from build123d import *

# Parameters (mm, degrees)
SKETCH1_W           = 8.3
SKETCH1_H           = 14.6
BOSS_EXTRUDE1_DEPTH = 1.5
SKETCH2_R           = 1.7
CUT_EXTRUDE1_DEPTH  = 1.5
SKETCH3_W           = 2.7
SKETCH3_H           = 3.5
BOSS_EXTRUDE3_DEPTH = 1.5


with BuildPart() as part:
    # Sketch1 → Boss-Extrude1 (new body)
    with BuildSketch(Plane.XY):
        with Locations((4.15, 7.3)):
            Rectangle(SKETCH1_W, SKETCH1_H)
    extrude(amount=BOSS_EXTRUDE1_DEPTH)

    # Sketch2 → Cut-Extrude1 (cut)
    with BuildSketch(Plane.XY.offset(1.5)):
        with Locations((4.15, 11.6)):
            Circle(SKETCH2_R)
    extrude(amount=-CUT_EXTRUDE1_DEPTH, mode=Mode.SUBTRACT)

    # Sketch3 → Boss-Extrude3 (add)
    with BuildSketch(Plane.XY.offset(1.5)):
        with Locations((4.15, 6.85)):
            Rectangle(SKETCH3_W, SKETCH3_H)
    extrude(amount=BOSS_EXTRUDE3_DEPTH)


solid = part.part
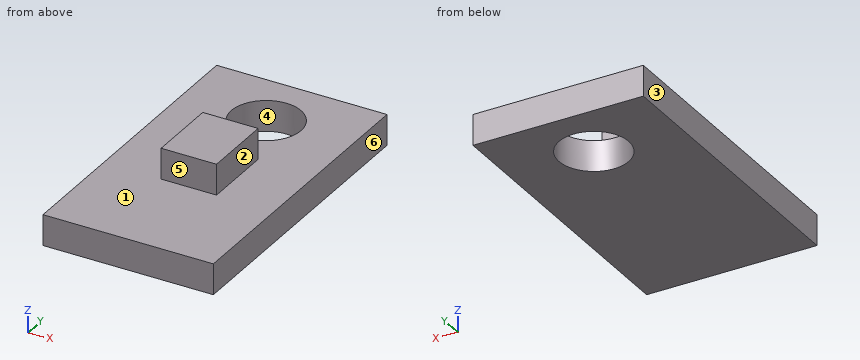
Verification items for the finished model (mm, model axes). Face numbers are marked on the shaded views. A direction names the side the tool comes from. Give positions to 0.01 mm unless a question says otherwise; leave off trailing zeros. Loops run counter-clockwise (first coordinate to the right, second up) from the corner with the lowest first, then second, coordinate; pieces in that order, holes last.
1) Thickness scan on line 1 along Y through (x, z) = (4.15, 0.9); line 2 along Z through (x, y) = (7.5, 3.25); line 3 along X through (y, z) = (7.25, 1.95). Record the ranges inside material, lowest first.
2) Sectioned sample at A-A, the plane x = 4.15. Enter the section's corners in (y, z), then the cut area to 4 significant figures.
3) Draft check along X on the marked faces 1, 2, 3 and 4. Enter one of: pulls with the +X half, pulls with the -X half, needs draft (parallel to the pull), parting line crosses it, or undercut.
4) Sectioned sample at C-C, the plane z = 0.8. Enter the section's corners in (x, y), then the cut area to 3 significant figures.
5) Set-up check for the marked faces 5 and 6: record each of +Z, -Z, +X, -X, +Y, -Y from which the full face is reachable in a straight line by a thin tool's end or side.
6) Sectioned sample at B-B, the plane y = 11.6. Enter the section's corners in (x, z), then the cut area to 3 significant figures.
7) Sectioned sample at D-D, the plane y = 8.25. Enter the section's corners in (x, z), then the cut area to 3 significant figures.
8) Depth check by flat-ended pin: pin 1 Ø1.5 at (x, z) = (2.5, 2.5) entering from -Y; pin 2 Ø1 at (x, y) = (4.5, 3) entering from +Z. Enter the tip coordinate at first touch or a pass-through.
Answers:
1. line 1: y = 0 to 9.9, 13.3 to 14.6
1. line 2: z = 0 to 1.5
1. line 3: x = 2.8 to 5.5
2. outline: (0, 0) - (9.9, 0) - (9.9, 1.5) - (8.6, 1.5) - (8.6, 3) - (5.1, 3) - (5.1, 1.5) - (0, 1.5) - close; (13.3, 0) - (14.6, 0) - (14.6, 1.5) - (13.3, 1.5) - close
2. area: 22.05 mm2
3. face 1: needs draft
3. face 2: pulls with the +X half
3. face 3: pulls with the -X half
3. face 4: undercut
4. outline: (0, 0) - (8.3, 0) - (8.3, 14.6) - (0, 14.6) - close; hole circle Ø3.4 at (4.15, 11.6)
4. area: 112 mm2
5. face 5: +Z, +X, -X, -Y
5. face 6: +Z, -Z, +X, +Y, -Y
6. outline: (0, 0) - (2.45, 0) - (2.45, 1.5) - (0, 1.5) - close; (5.85, 0) - (8.3, 0) - (8.3, 1.5) - (5.85, 1.5) - close
6. area: 7.35 mm2
7. outline: (0, 0) - (8.3, 0) - (8.3, 1.5) - (5.5, 1.5) - (5.5, 3) - (2.8, 3) - (2.8, 1.5) - (0, 1.5) - close
7. area: 16.5 mm2
8. pin 1: stops at y = 5.1
8. pin 2: stops at z = 1.5
